from build123d import *

# Parameters (mm, degrees)
F3_DEPTH      = 61.9125
F5_DEPTH      = 50.8
F5_DEPTH_BACK = 3.175
F7_DEPTH      = 967.58125


with BuildPart() as f3:
    # F2 (on offset) → F3 (new body)
    with BuildSketch(Plane.XZ.offset(-3.175)):
        Polygon((0, 2085.975), (0, 0), (19.05, 0), (31.75, 0), (31.75, 2073.275), (935.83125, 2073.275), (935.83125, 0), (948.53125, 0), (967.58125, 0), (967.58125, 2105.025), (0, 2105.025), align=None)
    extrude(amount=-F3_DEPTH)

    # F4 (on Front) → F5 (join, two sides)
    with BuildSketch(Plane.XZ) as f5_sk:
        Polygon((0, 2085.975), (0, 0), (19.05, 0), (19.05, 2073.275), (19.05, 2085.975), (948.53125, 2085.975), (948.53125, 0), (967.58125, 0), (967.58125, 2105.025), (0, 2105.025), align=None)
    extrude(amount=F5_DEPTH)
    extrude(f5_sk.sketch, amount=-F5_DEPTH_BACK)

    # F6 (on Right) → F7 (join, through all)
    with BuildSketch(Plane.YZ):
        Polygon((32.54375, 12.7), (-18.25625, 12.7), (-56.35625, 0), (-50.8, 0), (7.14375, 0), (65.0875, 0), (70.64375, 0), align=None)
    extrude(amount=F7_DEPTH)


solid = f3.part
Here's how the part is built. I have some questions about the finished solid (model axes, mm). A direction names the side the tool comes from. Round coordinates to 2 decimals unless told otherwise and drop trailing zeros. Order: outer loops, then holes, each group sorted by start corner. A loop starts at its lowest first (then second) coordinate and runs counter-clockwise, first axis right, second up. Notation, with made-up numbers: M 23,56.5 L 30,56.5 A15 cw 30,83.5 Z; hole C -7,-12.5 d4. An arc over 180 degrees is marked long. Return JSON: item names as keys, results as strings. Group by question number.
1. If we mould it in two halves opening along Z, with no side actions, what happens to faces 1 (the face through (477, -24, 2085.975)), 2 (the face through (16, 65.088, 1058)), 3 (the face through (477, 6, 0))? For each: pulls with the +Z half, pulls with the -Z half, needs draft (parallel to the pull), parting line crosses it, or undercut.
2. On a 3-axis mill with a long thin cutter (end or side, diameter ignored), from which of +Z, -Z, +X, -X, +Y, -Y can I reach the whole of each face in a straight line? I mean faces 4 (the face through (477.02, -37.04, 6.44)), 5 (the face through (477, 34, 2073.275)), 6 (the face through (16, -50.8, 1058)). Say none if no direction works.
3. Please list where these lines run through material, in increasing order: probe 1 along X at (y, z) = (38, 1938); probe 2 along Z at (x, y) = (744, 13.5) (3 decimals); probe 3 along Z at (x, y) = (124, -8) (3 decimals).
4. If we section it at B-B on x = 866.5: List the corners of the cut face in (y, z) for me (1 decimal).
Reply:
{
 "1": {"face 1": "undercut", "face 2": "needs draft", "face 3": "pulls with the -Z half"},
 "2": {"face 4": "-Y", "face 5": "+Y, -Y", "face 6": "+Z, +X, -X, -Y"},
 "3": {"probe 1": "0 to 31.75, 935.83 to 967.58", "probe 2": "0 to 12.7, 2073.275 to 2105.025", "probe 3": "0 to 12.7, 2085.975 to 2105.025"},
 "4": {"outline": "M -56.4,0 L 70.6,0 L 32.5,12.7 L -18.3,12.7 Z; M -50.8,2086 L 3.2,2086 L 3.2,2073.3 L 65.1,2073.3 L 65.1,2105 L -50.8,2105 Z"}
}
